The model under review builds one solid part; all positions refer to its coordinate system, in mm. A direction names the side the tool comes from. Coordinates: 2 decimals unless noted, no trailing zeros. Loops run counter-clockwise (first coordinate to the right, second up) from the corner with the lowest first, then second, coordinate; pieces in that order, holes last. Notation, with made-up numbers: M 31,-38.5 L 35,-38.5 A20 cw 35,-15.5 Z; hole C -16,5 d10. An arc over 180 degrees is marked long. Use one line per item in the form item = value.
```python
from build123d import *

# Parameters (mm, degrees)
SKETCH1_R               = 10
BOSS_EXTRUDE1_DEPTH     = 25
SKETCH1_3_R             = 5
CUT_EXTRUDE2_DEPTH      = 26
CUT_EXTRUDE2_DEPTH_BACK = 25
SKETCH1_7_R             = 10
SKETCH1_7_R_2           = 7
SKETCH1_7_R_3           = 5
CUT_EXTRUDE3_DEPTH      = 2
SKETCH5_R               = 8
CUT_EXTRUDE4_DEPTH      = 2
SKETCH6_R               = 1.3
BOSS_EXTRUDE2_DEPTH     = 2
FILLET1_R               = 2
FILLET2_R               = 0.5


with BuildPart() as part:
    # Sketch1 → Boss-Extrude1 (new body)
    with BuildSketch(Plane.XY):
        Circle(SKETCH1_R)
    extrude(amount=BOSS_EXTRUDE1_DEPTH)

    # Sketch1<3> → Cut-Extrude2 (cut, two sides)
    with BuildSketch(Plane.XY) as cut_extrude2_sk:
        Circle(SKETCH1_3_R)
    extrude(amount=CUT_EXTRUDE2_DEPTH, mode=Mode.SUBTRACT)
    extrude(cut_extrude2_sk.sketch, amount=-CUT_EXTRUDE2_DEPTH_BACK, mode=Mode.SUBTRACT)

    # Sketch1<7> → Cut-Extrude3 (cut)
    with BuildSketch(Plane.XY):
        Circle(SKETCH1_7_R)
        Circle(SKETCH1_7_R_2, mode=Mode.SUBTRACT)
        Circle(SKETCH1_7_R_3)
    extrude(amount=CUT_EXTRUDE3_DEPTH, mode=Mode.SUBTRACT)

    # Sketch5 → Cut-Extrude4 (cut)
    with BuildSketch(Plane.XY.offset(25)):
        Circle(SKETCH5_R)
    extrude(amount=-CUT_EXTRUDE4_DEPTH, mode=Mode.SUBTRACT)

    # Sketch6 → Boss-Extrude2 (add)
    with BuildSketch(Plane.XY.offset(25)):
        with BuildLine():
            Line((-14.222467655, 1), (-14.222467655, -1))
            ThreePointArc((-14.222467655, -1), (-13.636681217, -2.414213562), (-12.222467655, -3))
            Line((-12.222467655, -3), (-9.539392014, -3))
            ThreePointArc((-9.539392014, -3), (-10, 0), (-9.539392014, 3))
            Line((-9.539392014, 3), (-12.222467655, 3))
            ThreePointArc((-12.222467655, 3), (-13.636681217, 2.414213562), (-14.222467655, 1))
        make_face()
        with Locations((-12, 0)):
            Circle(SKETCH6_R, mode=Mode.SUBTRACT)
        with BuildLine():
            ThreePointArc((10, 0), (9.884177258, -1.517576993), (9.539392014, -3))
            Line((9.539392014, -3), (12.222467655, -3))
            ThreePointArc((12.222467655, -3), (13.636681217, -2.414213562), (14.222467655, -1))
            Line((14.222467655, -1), (14.222467655, 1))
            ThreePointArc((14.222467655, 1), (13.636681217, 2.414213562), (12.222467655, 3))
            Line((12.222467655, 3), (9.539392014, 3))
            ThreePointArc((9.539392014, 3), (9.884177258, 1.517576993), (10, 0))
        make_face()
        with Locations((12, 0)):
            Circle(SKETCH6_R, mode=Mode.SUBTRACT)
    extrude(amount=-BOSS_EXTRUDE2_DEPTH)

    # Fillet1
    fillet1_edges = [part.edges().sort_by_distance(p)[0] for p in [
        (-10, 0, 2),
    ]]
    fillet(fillet1_edges, radius=FILLET1_R)

    # Fillet2
    fillet2_edges = [part.edges().sort_by_distance(p)[0] for p in [
        (-7, 0, 2),
        (-7, 0, 0),
        (-13.636681217, 2.414213562, 23),
        (-10.880929834, -3, 23),
        (-13.636681217, -2.414213562, 23),
        (-14.222467655, 0, 23),
        (-10.880929834, 3, 23),
        (14.222467655, 0, 23),
        (13.636681217, -2.414213562, 23),
        (10.880929834, 3, 23),
        (13.636681217, 2.414213562, 23),
        (10.880929834, -3, 23),
    ]]
    fillet(fillet2_edges, radius=FILLET2_R)


solid = part.part
```
1. Wall thickness on line 1 along X through (y, z) = (0.25, 10); line 2 along Y through (x, z) = (0, 6.25); line 3 along Y through (x, z) = (0, 23.6): over which ranges is each line inside the solid? List them lowest first. Write a range as from..to.
Response values:
line_1 = -10..-4.99, 4.99..10
line_2 = -10..-5, 5..10
line_3 = -10..-8, 8..10
2. Machinability: for faces 1 (the face through (-11, -3, 24)), 2 (the face through (-1.73, -7.81, 24.01)), 3 (the face through (-11, 3, 24)), 4 (the face through (5, -6, 2)), 5 (the face through (11, 3, 24)), which of the approach directions +Z, -Z, +X, -X, +Y, -Y give a long, thin tool a straight path to every point of the face, cutting with its end or side? Answer none if there is none.
Response values:
face_1 = +Z, -Z, -X, -Y
face_2 = +Z
face_3 = +Z, -Z, -X, +Y
face_4 = -Z
face_5 = +Z, -Z, +X, +Y
3. Add section A-A (x = 0). State the section outline as (y, z) points.
Response values:
outline = M -10,4 A2 ccw -8,2 L -7.5,2 A0.5 cw -7,1.5 L -7,0.5 A0.5 ccw -6.5,0 L -5,0 L -5,23 L -8,23 L -8,25 L -10,25 Z; M 5,0 L 6.5,0 A0.5 ccw 7,0.5 L 7,1.5 A0.5 cw 7.5,2 L 8,2 A2 ccw 10,4 L 10,25 L 8,25 L 8,23 L 5,23 Z
4. Add section C-C (y = 0). Count the separate pieces of the cut face and the enclosed holes in it, then the cut area to 3 significant figures.
Response values:
separate_pieces = 4
enclosed_holes = 0
area = 231 mm^2
5. Insertion check: P1, Ø0.8, axis at x = -10.5, z = 24.5, coming from the +Y side; P2, Ø8, axis at y = -4, z = 16.5, coming from the +X side; P3, Ø5, axis at y = 1, z = 6.5, coming from the -X side. Each pin has a flat end and moves straight along its axis. Give the tip position at first contact, or say it passes through.
Response values:
P1 = 3
P2 = 10
P3 = -10
6. Add section B-B (z = 21.5). State the section outline as (x, y) points, then the cut area to 3 significant figures.
Response values:
outline = C 0,0 d20; hole C 0,0 d10
area = 236 mm^2
7. The part is to be moulded in two halves that separate along X. For faces 6 (the face through (9.237, -3.83, 14.353)), 7 (the face through (11, -3, 24)), 8 (the face through (-10.76, 0.39, 24.01)), say which applies: pulls with the +X half, pulls with the -X half, needs draft (parallel to the pull), parting line crosses it, or undercut.
Response values:
face_6 = parting line crosses it
face_7 = needs draft
face_8 = undercut
